Model file for the job. Use its own axes, mm. A direction names the side the tool comes from. Coordinates: 2 decimals unless noted, no trailing zeros. Order: outer loops, then holes, each group sorted by start corner. A loop starts at its lowest first (then second) coordinate and runs counter-clockwise, first axis right, second up.
from build123d import *

# Parameters (mm, degrees)
SKETCH1_R           = 6.35
BOSS_EXTRUDE1_DEPTH = 104.775
SKETCH3_R           = 3.175
CUT_EXTRUDE1_DEPTH  = 19.05
SKETCH2_R           = 3.175
CUT_EXTRUDE2_DEPTH  = 19.05


with BuildPart() as part:
    # Sketch1 → Boss-Extrude1 (new body, symmetric)
    with BuildSketch(Plane.XY):
        Circle(SKETCH1_R)
    extrude(amount=BOSS_EXTRUDE1_DEPTH, both=True)

    # Sketch3 → Cut-Extrude1 (cut)
    with BuildSketch(Plane(origin=(0, 0, -104.775), x_dir=(-1, 0, 0), z_dir=(0, 0, -1))):
        Circle(SKETCH3_R)
    extrude(amount=-CUT_EXTRUDE1_DEPTH, mode=Mode.SUBTRACT)

    # Sketch2 → Cut-Extrude2 (cut)
    with BuildSketch(Plane.XY.offset(104.775)):
        Circle(SKETCH2_R)
    extrude(amount=-CUT_EXTRUDE2_DEPTH, mode=Mode.SUBTRACT)


solid = part.part
Q1. Drop flat-ended pins along their axis: P1, Ø7.5, axis at x = 0, y = 0, coming from the -Z side (3 decimals); P2, Ø5, axis at y = -3.5, z = -7.5, coming from the +X side; P3, Ø4, axis at x = 0, y = 0, coming from the -Z side (3 decimals); P4, Ø4, axis at y = -4, z = -41.5, coming from the -X side. Give the stop position or say it passes through.
Established:
P1: stops at z = -104.775
P2: stops at x = 6.27
P3: stops at z = -85.725
P4: stops at x = -6.03
Q2. Which spindle directions (+Z, -Z, +X, -X, +Y, -Y) get a long thin tool onto all of the face, cutting with end or side? Do faces 4 (the face through (-2, 3, 104.775)), 5 (the face through (0, 0, 85.725)), 6 (the face through (0, 0, -85.725)). Say none if no direction does.
Established:
face 4: +Z, +X, -X, +Y, -Y
face 5: +Z
face 6: -Z
Q3. Cut at C-C, the plane z = 61.5. List the corners of the cut face in (x, y), plus the area to 3 significant figures.
Established:
outline: circle Ø12.7 at (0, 0)
area: 127 mm2
Q4. Mould opens along Y. For faces 1 (the face through (0.69, -3.1, -95.38)), 2 (the face through (-1.38, -6.2, 1.47)), 3 (the face through (-2, 3, -104.775)) say: pulls with the +Y half, pulls with the -Y half, needs draft (parallel to the pull), parting line crosses it, or undercut.
Established:
face 1: undercut
face 2: parting line crosses it
face 3: needs draft
Q5. Probe line 1 (Y direction, x = 0, z = -92) (3 decimals); line 2 (Z direction, x = -1.25, y = -2.5) (3 decimals); line 3 (Y direction, x = -0.25, z = 3). List the from-to ranges inside material, lowest first.
Established:
line 1: y = -6.35 to -3.175, 3.175 to 6.35
line 2: z = -85.725 to 85.725
line 3: y = -6.35 to 6.35
Q6. Cut at A-A, the plane x = 0. List the corners of the cut face in (y, z) (3 decimals), plus the area to 3 significant figures.
Established:
outline: (-6.35, -104.775) - (-3.175, -104.775) - (-3.175, -85.725) - (3.175, -85.725) - (3.175, -104.775) - (6.35, -104.775) - (6.35, 104.775) - (3.175, 104.775) - (3.175, 85.725) - (-3.175, 85.725) - (-3.175, 104.775) - (-6.35, 104.775) - close
area: 2,420 mm2
